```python
from build123d import *

# Parameters (mm, degrees)
F0_W          = 2.54
F0_H          = 2.54
F1_DEPTH      = 21.59
F3_DEPTH      = 2.54
F3_DEPTH_BACK = 2.54
F5_DEPTH      = 12.7
F7_DEPTH      = 25.4
F8_R          = 1.26999


# Not quite as in the source:
# - a fillet or chamfer is up to 0.001 mm smaller than in the source, because OpenCascade refuses the exact size


with BuildPart() as f1:
    # F0 (on Front) → F1 (new body)
    with BuildSketch(Plane.XZ):
        with Locations((1.27, 1.27)):
            Rectangle(F0_W, F0_H)
    extrude(amount=F1_DEPTH)

    # F2 (on face) → F3 (join, two sides)
    with BuildSketch(Plane.YZ.offset(2.54)) as f3_sk:
        Polygon((-18.415, 8.89), (-18.415, 2.54), (-18.415, 0), (-3.175, 0), (-3.175, 2.54), (-3.175, 8.89), align=None)
    extrude(amount=F3_DEPTH)
    extrude(f3_sk.sketch, amount=-F3_DEPTH_BACK)

    # F4 (on face) → F5 (join)
    with BuildSketch(Plane.YZ.offset(5.08)):
        Polygon((-18.415, 8.89), (-18.415, 0), (-15.24, 0), (-15.24, 6.35), (-6.35, 6.35), (-6.35, 0), (-3.175, 0), (-3.175, 8.89), align=None)
    extrude(amount=F5_DEPTH)

    # F6 (on face) → F7 (cut)
    with BuildSketch(Plane(origin=(0, 0, 6.35), x_dir=(1, 0, 0), z_dir=(0, 0, -1))):
        with BuildLine():
            ThreePointArc((12.8865943547, 11.8146160483), (10.4103839517, 12.2515943547), (9.9734056453, 9.7753839517))
            Line((9.9734056453, 9.7753839517), (12.8865943547, 11.8146160483))
        make_face()
        with BuildLine():
            Line((12.8865943547, 11.8146160483), (9.9734056453, 9.7753839517))
            ThreePointArc((9.9734056453, 9.7753839517), (11.9645368263, 9.099254034), (13.208, 10.795))
            ThreePointArc((13.208, 10.795), (13.125745966, 11.3295368263), (12.8865943547, 11.8146160483))
        make_face()
    extrude(amount=-F7_DEPTH, mode=Mode.SUBTRACT)

    # F8 (radius 1.27 in the source; OpenCascade refuses exactly that, so slightly less here)
    f8_edges = [f1.edges().sort_by_distance(p)[0] for p in [
        (0, -1.5875, 2.54),
        (2.54, -1.5875, 2.54),
        (0, -20.0025, 2.54),
        (2.54, -20.0025, 2.54),
    ]]
    fillet(f8_edges, radius=F8_R)


solid = f1.part
```
The model under review builds one solid part; all positions refer to its coordinate system, in mm. A direction names the side the tool comes from. Coordinates: 2 decimals unless noted, no trailing zeros. Write each loop counter-clockwise with the first axis right and the second up, starting at its lowest first coordinate (ties: lowest second). Pieces come first, ordered by that corner, then holes. Notation, with made-up numbers: (-11, 5.5) - (39, 5.5) arc R3 ccw to (39, 9.5) - close; hole circle Ø3 at (36.25, -13.75). An arc over 180 degrees is marked (long way). Answer in a Markdown table with one row per item. Add a question column.
Q1. For faces 1 (the face through (11, -13, 6.35)), 2 (the face through (2.178, -20.025, 2.158)), 3 (the face through (0.362, -1.61, 2.158)), 4 (the face through (0.382, -20.025, 2.178)), 5 (the face through (2.54, -2, 1)), list the 3-axis set-ups (+Z, -Z, +X, -X, +Y, -Y) from which the entire face can be reached by the end or side of a thin tool; tool diameter is ignored.
Q2. Consider section A-A on x = 11.43. Give the boundary of the cut face in (y, z) (3 decimals).
Q3. Consider section B-B on z = 7. Give the boundary of the cut face in (x, y) (3 decimals), then the cut area to 3 significant figures.
Q4. Draft analysis for pull direction Y (two halves, no side actions). For faces 6 (the face through (1, -21.59, 1)), 7 (the face through (11, -15.24, 3)), 8 (the face through (1, 0, 1)), 9 (the face through (2.54, -20, 1)), state which applies: +Y half, -Y half, draft (parallel to the pull), parting line (faces both ways), or undercut.
Q5. Consider section D-D on y = -7.25. Give the boundary of the cut face in (x, z), then the cut area to 3 significant figures.
Q6. To check wall thickness, follow line 1 along Y through (x, z) = (15.75, 2.75) (3 decimals); line 2 along Y through (x, z) = (8, 7) (3 decimals); line 3 along X through (y, z) = (-13.75, 1.25). State the ranges of each line that lie inside material, in increasing order. Write a range as from..to.
Q7. Clearance check with flat-ended pins moving along their axes: pin 1 (10 mm diameter, centred on x = 12, y = -10, fed in from -Z); pin 2 (1.5 mm diameter, centred on x = 3.5, z = 4, fed in from -Y) (3 decimals); pin 3 (1.4 mm diameter, centred on y = -1, z = 1, fed in from +X); pin 4 (1.9 mm diameter, centred on y = -10.5, z = 4, fed in from +X). State where each tip first meets the part, or that it passes through.
Q8. Consider section C-C on y = -11.5. Give the boundary of the cut face in (x, z).
Answers below:
| question | item | result |
|---|---|---|
| 1 | face 1 | -Z, +X |
| 1 | face 2 | +Z, +X, -Y |
| 1 | face 3 | +Z, -X, +Y |
| 1 | face 4 | +Z, -X, -Y |
| 1 | face 5 | +Z, -Z, +X, +Y |
| 2 | outline | (-18.415, 0) - (-15.24, 0) - (-15.24, 6.35) - (-12.573, 6.35) - (-12.573, 8.89) - (-18.415, 8.89) - close; (-9.017, 6.35) - (-6.35, 6.35) - (-6.35, 0) - (-3.175, 0) - (-3.175, 8.89) - (-9.017, 8.89) - close |
| 3 | outline | (0, -18.415) - (17.78, -18.415) - (17.78, -3.175) - (0, -3.175) - close; hole circle Ø3.556 at (11.43, -10.795) |
| 3 | area | 261 mm² |
| 4 | face 6 | -Y half |
| 4 | face 7 | undercut |
| 4 | face 8 | +Y half |
| 4 | face 9 | draft |
| 5 | outline | (0, 0) - (5.08, 0) - (5.08, 6.35) - (17.78, 6.35) - (17.78, 8.89) - (0, 8.89) - close |
| 5 | area | 77.4 mm² |
| 6 | line 1 | -18.415..-15.24, -6.35..-3.175 |
| 6 | line 2 | -18.415..-3.175 |
| 6 | line 3 | 0..5.08 |
| 7 | pin 1 | z = 0 |
| 7 | pin 2 | y = -18.415 |
| 7 | pin 3 | x = 2.54 |
| 7 | pin 4 | x = 5.08 |
| 8 | outline | (0, 0) - (5.08, 0) - (5.08, 6.35) - (9.8, 6.35) - (9.8, 8.89) - (0, 8.89) - close; (13.06, 6.35) - (17.78, 6.35) - (17.78, 8.89) - (13.06, 8.89) - close |
